Geometry check sheet. Reference: the model listing, model coordinates, mm. A direction names the side the tool comes from. Round coordinates to 2 decimals unless told otherwise and drop trailing zeros. Order: outer loops, then holes, each group sorted by start corner. A loop starts at its lowest first (then second) coordinate and runs counter-clockwise, first axis right, second up. Notation, with made-up numbers: (-10, 81.5) -> (40, 81.5) arc R24 cw to (40, 104.5) -> close; hole circle Ø1 at (-27.5, -17.5). An arc over 180 degrees is marked (long way). Use a Markdown table: item, result. Add a question column.
Item 1: Sectioned sample at B-B, the plane z = 0. Record the cut outline in (x, y), and give its area (3 significant figures).
Item 2: Gauge pin test, flat ends, axial feed: pin 1 Ø2 at (x, y) = (3, 2.5) entering from -Z; pin 2 Ø1 at (x, y) = (3, 2) entering from -Z. Record the tip position at first contact, or that the pin passes through.
Item 3: Sectioned sample at A-A, the plane x = 0. Record the cut outline in (y, z).
Item 4: Sectioned sample at C-C, the plane y = 2. Record the cut outline in (x, z), and give its area (3 significant figures).
Item 5: Set-up check for faces 1 (the flat face through (2, 0, 3)), 2 (the flat face through (-3, 1, -1)): record each of +Z, -Z, +X, -X, +Y, -Y from which the full face is reachable in a straight line by a thin tool's end or side.
Item 6: Material ranges on probe 1 along X at (y, z) = (2.8, 0); probe 2 along Z at (x, y) = (0, 0.75), recorded low to high. Write a range as [from, to].
from build123d import *

# Parameters (mm, degrees)
SKETCH1_R           = 5
SKETCH1_R_2         = 3.5
BOSS_EXTRUDE1_DEPTH = 4
SKETCH2_R           = 5
SKETCH2_R_2         = 2.75
BOSS_EXTRUDE2_DEPTH = 1
CHAMFER1_SIZE       = 0.2
CHAMFER2_SIZE       = 0.6


with BuildPart() as part:
    # Sketch1 → Boss-Extrude1 (new body)
    with BuildSketch(Plane(origin=(0, 0, 0), x_dir=(1, 0, 0), z_dir=(0, 1, 0))):
        Circle(SKETCH1_R)
        Circle(SKETCH1_R_2, mode=Mode.SUBTRACT)
    extrude(amount=BOSS_EXTRUDE1_DEPTH)

    # Sketch2 → Boss-Extrude2 (add)
    with BuildSketch(Plane.XZ):
        Circle(SKETCH2_R)
        Circle(SKETCH2_R_2, mode=Mode.SUBTRACT)
    extrude(amount=-BOSS_EXTRUDE2_DEPTH)

    # Chamfer1
    chamfer1_edges = [part.edges().sort_by_distance(p)[0] for p in [
        (-2.75, 1, 0),
        (-5, 0, 0),
        (-5, 4, 0),
        (-3.5, 4, 0),
    ]]
    chamfer(chamfer1_edges, length=CHAMFER1_SIZE)

    # Chamfer2
    chamfer2_edges = [part.edges().sort_by_distance(p)[0] for p in [
        (-2.75, 0, 0),
    ]]
    chamfer(chamfer2_edges, length=CHAMFER2_SIZE)


solid = part.part
Found:
| question | item | result |
|---|---|---|
| 1 | outline | (-5, 0.2) -> (-4.8, 0) -> (-3.35, 0) -> (-2.75, 0.6) -> (-2.75, 0.8) -> (-2.95, 1) -> (-3.5, 1) -> (-3.5, 3.8) -> (-3.7, 4) -> (-4.8, 4) -> (-5, 3.8) -> close; (2.75, 0.6) -> (3.35, 0) -> (4.8, 0) -> (5, 0.2) -> (5, 3.8) -> (4.8, 4) -> (3.7, 4) -> (3.5, 3.8) -> (3.5, 1) -> (2.95, 1) -> (2.75, 0.8) -> close |
| 1 | area | 13.0 mm2 |
| 2 | pin 1 | stops at z = -4.58 |
| 2 | pin 2 | stops at z = -4.33 |
| 3 | outline | (0, -4.8) -> (0.2, -5) -> (3.8, -5) -> (4, -4.8) -> (4, -3.7) -> (3.8, -3.5) -> (1, -3.5) -> (1, -2.95) -> (0.8, -2.75) -> (0.6, -2.75) -> (0, -3.35) -> close; (0, 3.35) -> (0.6, 2.75) -> (0.8, 2.75) -> (1, 2.95) -> (1, 3.5) -> (3.8, 3.5) -> (4, 3.7) -> (4, 4.8) -> (3.8, 5) -> (0.2, 5) -> (0, 4.8) -> close |
| 4 | outline | circle Ø10 at (0, 0); hole circle Ø7 at (0, 0) |
| 4 | area | 40.1 mm2 |
| 5 | face 1 | +Z, -Z, +X, -X, -Y |
| 5 | face 2 | +Y |
| 6 | probe 1 | x = [-5, -3.5], [3.5, 5] |
| 6 | probe 2 | z = [-5, -2.75], [2.75, 5] |
